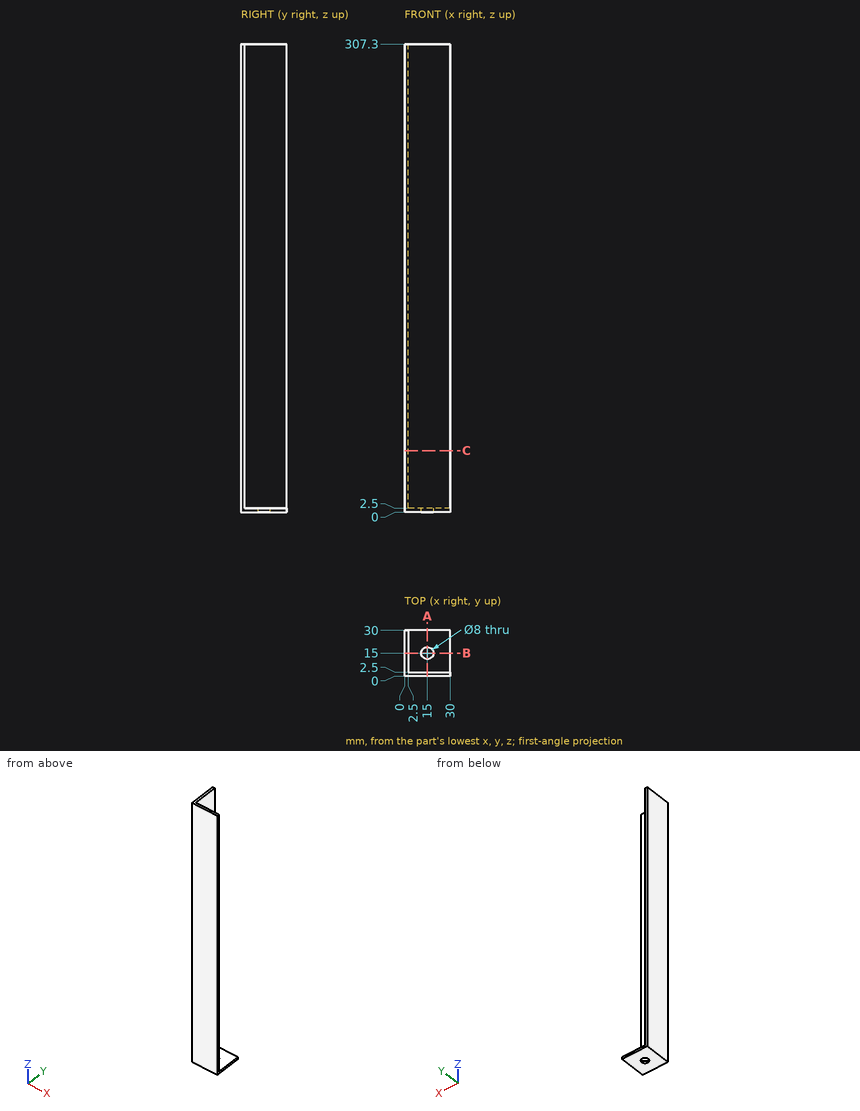
Check sheet for the drawn part. Datum: minimum x, y, z corner. Units: mm. Round coordinates to 2 decimals unless told otherwise and drop trailing zeros. Loops run counter-clockwise (first coordinate to the right, second up) from the corner with the lowest first, then second, coordinate; pieces in that order, holes last.
Item 1: Cross-section at C-C on z = 40.5. Record the boundary of the cut face in (x, y).
Item 2: Gauge pin test, flat ends, axial feed: pin 1 (1.5 mm diameter, centred on x = 7, z = 253, fed in from +Y); pin 2 (10 mm diameter, centred on y = 9, z = 71.5, fed in from -X); pin 3 (7 mm diameter, centred on x = 15, y = 15, fed in from +Z); pin 4 (2 mm diameter, centred on x = 17.5, y = 12, fed in from +Z). Record the tip position at first contact, or that the pin passes through.
Item 3: Thickness scan on line 1 (Y direction, x = 15, z = 1.25); line 2 (Z direction, x = 15.25, y = 28). Record the ranges inside material, lowest first.
Item 4: Cross-section at A-A on x = 15. Record the boundary of the cut face in (y, z), then the cut area to 3 significant figures.
Answer sheet:
1. outline: (0, 0) - (30, 0) - (30, 2.5) - (2.5, 2.5) - (2.5, 30) - (0, 30) - close
2. pin 1: stops at y = 2.5
2. pin 2: stops at x = 0
2. pin 3: passes through
2. pin 4: stops at z = 2.5
3. line 1: y = 0 to 11, 19 to 30
3. line 2: z = 0 to 2.5
4. outline: (0, 0) - (11, 0) - (11, 2.5) - (2.5, 2.5) - (2.5, 307.3) - (0, 307.3) - close; (19, 0) - (30, 0) - (30, 2.5) - (19, 2.5) - close
4. area: 817 mm2
